Verification items for this drawing (mm, ordinates from the low corner). A direction names the side the tool comes from. Give positions to 0.01 mm unless a question says otherwise; leave off trailing zeros. Loops run counter-clockwise (first coordinate to the right, second up) from the corner with the lowest first, then second, coordinate; pieces in that order, holes last. Notation, with made-up numbers: (9, 81.25) -> (68, 81.25) arc R10 ccw to (68, 98.25) -> close; hole circle Ø11 at (29, -4). An arc over 180 degrees is marked (long way). Write item = value, one per line.
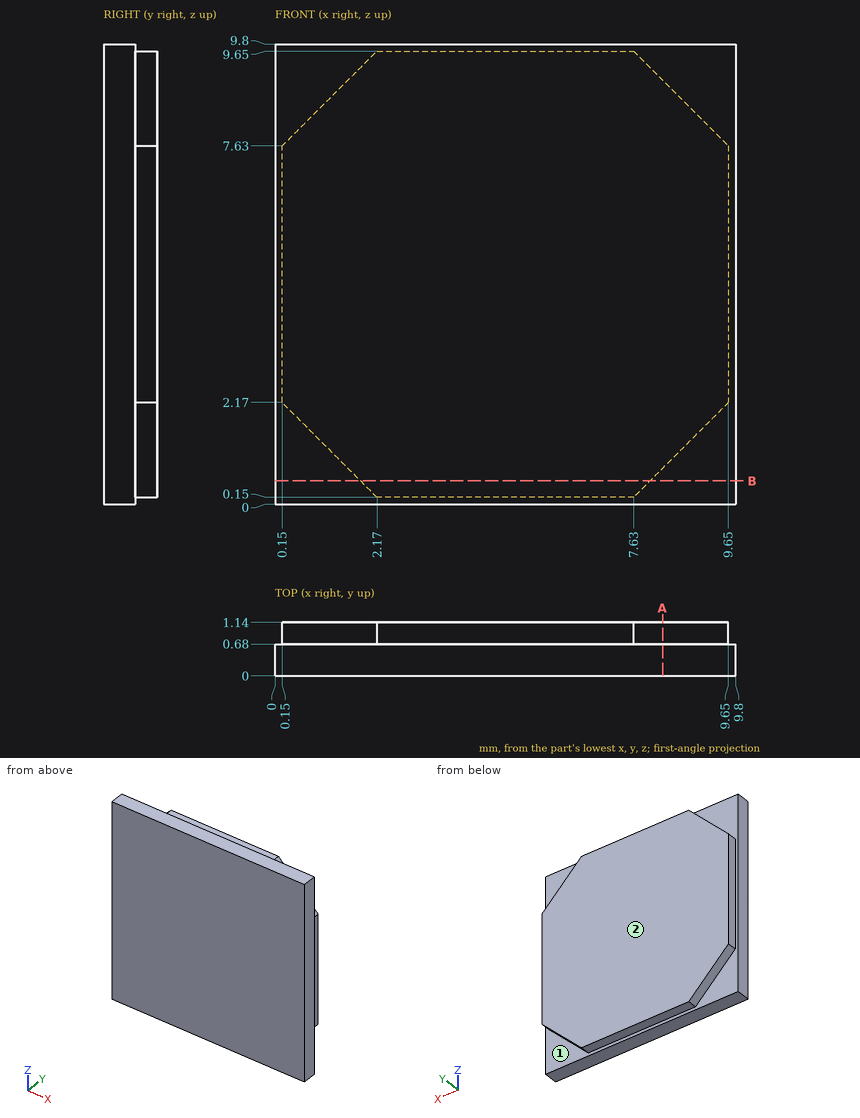
Item 1: Section check B-B, the plane z = 0.5. Record the cut outline in (x, y), plus the area to 3 significant figures.
Answer:
outline = (0, 0) -> (9.8, 0) -> (9.8, 0.68) -> (7.98, 0.68) -> (7.98, 1.14) -> (1.82, 1.14) -> (1.82, 0.68) -> (0, 0.68) -> close
area = 9.50 mm^2
Item 2: Thickness scan on L1, parallel to X at y = 0.9, z = 3.5; L2, parallel to Y at x = 0.5, z = 1. Record the ranges inside material, lowest first. Write a range as [from, to].
Answer:
L1 = [0.15, 9.65]
L2 = [0, 0.68]
Item 3: Gauge pin test, flat end, axial feed: pin 1 (0.5 mm diameter, centred on x = 4, y = 1, fed in from -Z). Record the tip position at first contact, or that the pin passes through.
Answer:
pin_1 = 0.15
Item 4: Tool access check on the marked faces 1 and 2. Record the directions out of +Z, -Z, +X, -X, +Y, -Y that give a thin tool (end or side, any length) a straight path to the whole face; none if there is none.
Answer:
face_1 = +Y
face_2 = +Z, -Z, +X, -X, +Y
Item 5: Section check A-A, the plane x = 8.25. Record the cut outline in (y, z).
Answer:
outline = (0, 0) -> (0.68, 0) -> (0.68, 0.77) -> (1.14, 0.77) -> (1.14, 9.03) -> (0.68, 9.03) -> (0.68, 9.8) -> (0, 9.8) -> close
